```python
from build123d import *

# Parameters (mm, degrees)
F0_W     = 186.055
F0_H     = 15.875
F1_DEPTH = 25.4
F2_R     = 7.93749
F4_D     = 9.525


# Not quite as in the source:
# - a fillet or chamfer is up to 0.001 mm smaller than in the source, because OpenCascade refuses the exact size


with BuildPart() as f1:
    # F0 (on Top) → F1 (new body)
    with BuildSketch(Plane.XY):
        Rectangle(F0_W, F0_H)
    extrude(amount=F1_DEPTH)

    # F2 (radius 7.9375 in the source; OpenCascade refuses exactly that, so slightly less here)
    f2_edges = [f1.edges().sort_by_distance(p)[0] for p in [
        (-93.0275, -7.9375, 12.7),
        (-93.0275, 7.9375, 12.7),
        (93.0275, -7.9375, 12.7),
        (93.0275, 7.9375, 12.7),
    ]]
    fillet(f2_edges, radius=F2_R)

    # F4 (through all)
    with Locations(Plane.XY.offset(25.4)):
        with Locations((-85.09, 0), (85.09, 0)):
            Hole(F4_D / 2)


solid = f1.part
```
The listing builds one solid part. Answer for the finished solid, in the listing's coordinates (mm). Give positions to 0.01 mm unless a question says otherwise; leave off trailing zeros. Write each loop counter-clockwise with the first axis right and the second up, starting at its lowest first coordinate (ties: lowest second). Pieces come first, ordered by that corner, then holes. Notation, with made-up numbers: (18, -15.75) - (59, -15.75) arc R26 cw to (59, 3.25) - close; hole circle Ø11 at (24.25, 77). An arc over 180 degrees is marked (long way). Use one line per item in the form item = value. Start each with the question number.
1) Find section A-A on z = 7.5. Count the separate pieces of the cut face and the enclosed holes in it, plus the area to 3 significant figures.
2) Flat-ended cylindrical pins translate along their axes: pin 1 Ø2 at (y, z) = (-0.5, 16.5) entering from -X; pin 2 Ø1 at (y, z) = (-3.5, 12.5) entering from +X; pin 3 Ø2 at (y, z) = (6, 14.5) entering from +X; pin 4 Ø5 at (y, z) = (4.5, 21.5) entering from -X. Find the tip coordinate at first contact, or state that the pin passes through.
3) Consider line 1 along X through (y, z) = (-3, 8.75); line 2 along X through (y, z) = (3.25, 20); line 3 along Y through (x, z) = (-84.5, 8). Determine where each line is inside the solid, lowest interval first. Write a range as from..to.
4) The mould has two halves that part along Y. Classify faces 1 (the face through (88.87, -2.9, 12.52)), 2 (the face through (-80.332, 0.209, 12.522)), 3 (the face through (-90.764, -5.551, 12.878)), 4 (the face through (90.764, 5.551, 12.878)): pulls with the +Y half, pulls with the -Y half, needs draft (parallel to the pull), parting line crosses it, or undercut.
5) Find section B-B on y = 1.75. Determine the outline of the cut face in (x, z), plus the area to 3 significant figures.
Geometry results:
q1.separate_pieces = 1
q1.enclosed_holes = 2
q1.area = 2,760 mm2
q2.pin_1 = -93.03
q2.pin_2 = 92.44
q2.pin_3 = 91.25
q2.pin_4 = -92.77
q3.line_1 = -92.44..-88.79, -81.39..81.39, 88.79..92.44
q3.line_2 = -92.33..-88.57, -81.61..81.61, 88.57..92.33
q3.line_3 = -7.94..-4.73, 4.73..7.94
q4.face_1 = undercut
q4.face_2 = undercut
q4.face_3 = pulls with the -Y half
q4.face_4 = pulls with the +Y half
q5.outline = (-92.83, 0) - (-89.52, 0) - (-89.52, 25.4) - (-92.83, 25.4) - close; (-80.66, 0) - (80.66, 0) - (80.66, 25.4) - (-80.66, 25.4) - close; (89.52, 0) - (92.83, 0) - (92.83, 25.4) - (89.52, 25.4) - close
q5.area = 4,270 mm2
